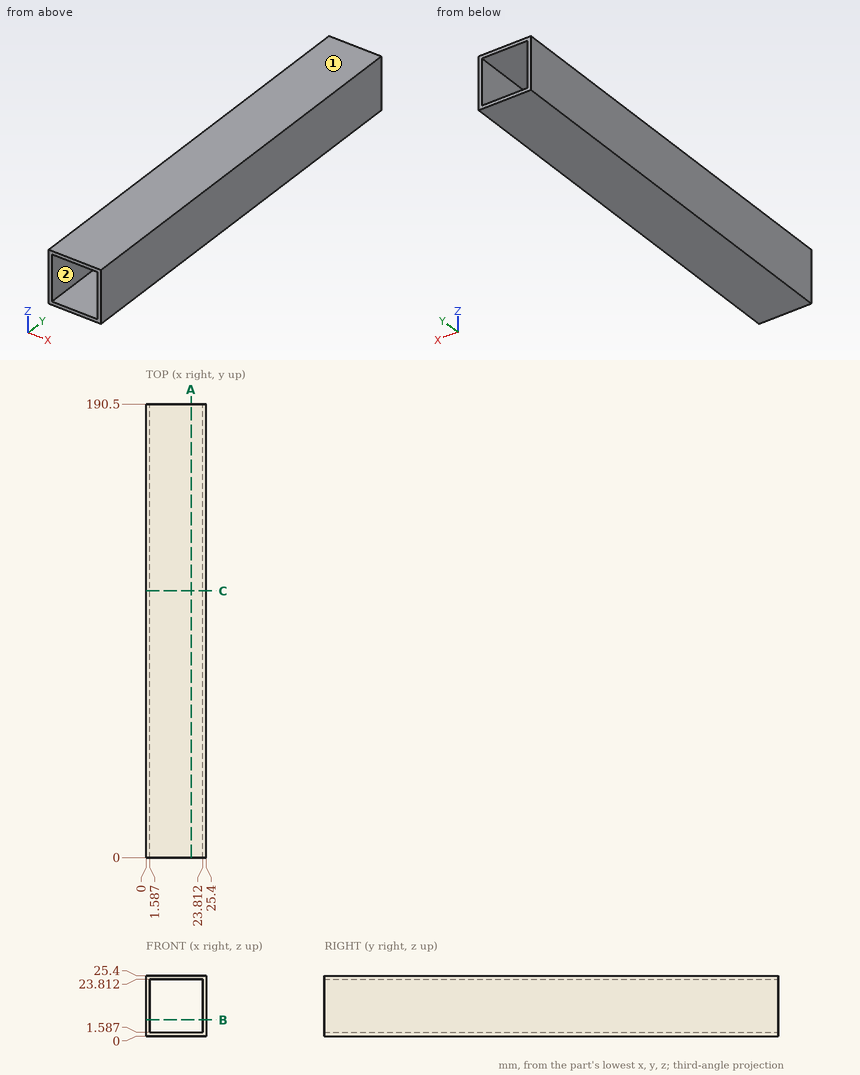
Geometry check sheet. Reference: drawing and pictorial views, mm from the part's lowest x, y, z. A direction names the side the tool comes from. Give positions to 0.01 mm unless a question says otherwise; leave off trailing zeros. Loops run counter-clockwise (first coordinate to the right, second up) from the corner with the lowest first, then second, coordinate; pieces in that order, holes last. Notation, with made-up numbers: (20.25, -6.5) - (50.25, -6.5) arc R11 ccw to (50.25, 7.5) - close; hole circle Ø9 at (78, 22). An arc over 180 degrees is marked (long way). Use CSV: the item, a comma, the result in double quotes. Start each with the question number.
Q1. Section check B-B, the plane z = 6.75. Record the cut outline in (x, y).
Q2. Section check A-A, the plane x = 19. Record the cut outline in (y, z).
Q3. Access from +Z, -Z, +X, -X, +Y, -Y to the whole of each face (thin tool, end or side, straight path). Record for the marked faces 1 and 2.
Q4. Go/stop test with a flat-tipped pin: pin 1 Ø4 at (x, z) = (8, 5.5) entering from +Y. Record where the tip stops, or that it passes through.
Q5. Scan line: probe 1 along Z at (x, y) = (6.5, 54.5). Record every from-to range of solid material in increasing order. Write a range as from..to.
Q6. Section check C-C, the plane y = 112. Record the cut outline in (x, z), and give its area (3 significant figures).
Findings below:
1,outline,"(0, 0) - (1.59, 0) - (1.59, 190.5) - (0, 190.5) - close; (23.81, 0) - (25.4, 0) - (25.4, 190.5) - (23.81, 190.5) - close"
2,outline,"(0, 0) - (190.5, 0) - (190.5, 1.59) - (0, 1.59) - close; (0, 23.81) - (190.5, 23.81) - (190.5, 25.4) - (0, 25.4) - close"
3,face 1,"+Z, +X, -X, +Y, -Y"
3,face 2,"+Y, -Y"
4,pin 1,"passes through"
5,probe 1,"z = 0..1.59, 23.81..25.4"
6,outline,"(0, 0) - (25.4, 0) - (25.4, 25.4) - (0, 25.4) - close; hole (1.59, 1.59) - (23.81, 1.59) - (23.81, 23.81) - (1.59, 23.81) - close"
6,area,"151 mm^2"
